Autodesk Inventor part; units mm, degrees
ref_plane "YZ Plane" through (0, 0, 0) normal (1, 0, 0) x (0, 1, 0)
ref_plane "XZ Plane" through (0, 0, 0) normal (0, 1, 0) x (-1, 0, 0)
ref_plane "XY Plane" through (0, 0, 0) normal (0, 0, 1) x (1, 0, 0)
sketch "Sketch1" plane through (0, 0, 0) normal (0, 0, 1) x (1, 0, 0)
  line L0 (0, 0) -> (150, 0)
  line L1 (150, 0) -> (150, 100)
  line L2 (150, 100) -> (0, 100)
  line L3 (0, 100) -> (0, 0)
  dimension "d0" = 150
  dimension "d1" = 100
extrude "Extrusion1" add sketch "Sketch1" along normal blind 250
fillet "Fillet1" radius 20 1 edges at (150, 100, 125)
fillet "Fillet2" radius 20 1 edges at (150, 0, 125)
fillet "Fillet3" radius 20 1 edges at (0, 100, 125)
fillet "Fillet4" radius 20 1 edges at (0, 0, 125)
fillet "Fillet5" radius 5 8 edges at (5.8579, 94.1421, 0) (0, 50, 0) (5.8579, 5.8579, 0) (75, 0, 0) (144.1421, 5.8579, 0) (150, 50, 0) (144.1421, 94.1421, 0) (75, 100, 0)
sketch "Sketch2" plane through (20, 0, 250) normal (0, -1, 0) x (1, 0, 0)
  line L0 (110, 0) -> (110, -245)
  line L1 (0, -245) -> (0, 0)
  line L2 (110, -171.6757) -> (0, -171.6757)
  line L3 (0, -171.6757) -> (0, -166.6757)
  line L4 (0, -166.6757) -> (110, -166.6757)
  line L5 (110, -166.6757) -> (110, -171.6757)
  line L6 (95.3863, -226.2308) -> (70.3863, -226.2308)
  line L7 (70.3863, -226.2308) -> (70.3863, -221.2308)
  line L8 (70.3863, -221.2308) -> (95.3863, -221.2308)
  line L9 (95.3863, -221.2308) -> (95.3863, -226.2308)
  line L10 (37.9599, -226.2308) -> (12.9599, -226.2308)
  line L11 (12.9599, -226.2308) -> (12.9599, -221.2308)
  line L12 (12.9599, -221.2308) -> (37.9599, -221.2308)
  line L13 (37.9599, -221.2308) -> (37.9599, -226.2308)
  line L14 (27.9599, -236.2308) -> (22.9599, -236.2308)
  line L15 (22.9599, -236.2308) -> (22.9599, -211.2308)
  line L16 (22.9599, -211.2308) -> (27.9599, -211.2308)
  line L17 (27.9599, -211.2308) -> (27.9599, -236.2308)
  point P0 (-20, -250)
  point P1 (27.9599, -226.2308)
  point P2 (27.9599, -221.2308)
  point P3 (22.9599, -221.2308)
  point P4 (22.9599, -226.2308)
  dimension "d9" = 25
  dimension "d10" = 5
  dimension "d11" = 5
  dimension "d12" = 25
  dimension "d13" = 10
  dimension "d14" = 10
  dimension "d15" = 5
  dimension "d16" = 25
  dimension "d17" = 5
extrude "Extrusion2" add sketch "Sketch2" along normal blind 5
sketch "Sketch3" plane through (0, 0, 0) normal (0, 0, -1) x (-1, 0, 0)
  line L0 (-20, 100) -> (-130, 100)
  line L1 (-150, 80) -> (-150, 20)
  circle A0 centre (-110, 50) radius 12.5
  circle A1 centre (-40, 51.4507) radius 12.5
  point P0 (0, 0)
  point P1 (-150, 50)
  dimension "d20" = 50
  dimension "d21" = 40
  dimension "d22" = 70
  dimension "d23" = 25
  dimension "d24" = 25
extrude "Extrusion3" add sketch "Sketch3" along normal blind 3
sketch "Sketch4" plane through (110, 50, -3) normal (0, 0, -1) x (-1, 0, 0)
  circle A0 centre (0, 0) radius 7.2404
  circle A1 centre (70, 1.4507) radius 12.5
  circle A2 centre (70, 1.4507) radius 7.5
  point P0 (110, -50)
  dimension "d27" = 15
extrude "Extrusion4" add sketch "Sketch4" along normal blind 15 contours A0 | A2
sketch "Sketch5" plane through (110, 50, -18) normal (0, 0, -1) x (-1, 0, 0)
  circle A0 centre (0, 0) radius 7.2404
  circle A1 centre (0, 0) radius 10
  circle A2 centre (70, 1.4507) radius 7.5
  circle A3 centre (70, 1.4507) radius 8.5
  point P0 (110, -50)
  dimension "d30" = 20
  dimension "d31" = 17
extrude "Extrusion5" add sketch "Sketch5" along normal blind 4 contours A0 | A1 | A2 | A3
sketch "Sketch6" plane through (110, 50, -22) normal (0, 0, -1) x (-1, 0, 0)
  circle A0 centre (0, 0) radius 10
  point P0 (110, -50)
hole "Hole1" at (110, 50, -22) direction (0, 0, 1) diameter 10.106 depth 28 tip angle 118
sketch "Sketch7" plane through (40, 51.4507, -22) normal (0, 0, -1) x (-1, 0, 0)
  circle A0 centre (0, 0) radius 8.5
  point P0 (40, -51.4507)
hole "Hole2" at (40, 51.4507, -22) direction (0, 0, 1) diameter 10.647 depth 28 tip angle 118
properties part number "battery eg 26"
The model under review builds one solid part; all positions refer to its coordinate system, in mm. A direction names the side the tool comes from. Coordinates: 2 decimals unless noted, no trailing zeros. Write each loop counter-clockwise with the first axis right and the second up, starting at its lowest first coordinate (ties: lowest second). Pieces come first, ordered by that corner, then holes.
1) Clearance check with flat-ended pins moving along their axes: pin 1 Ø8 at (x, z) = (68, 46.5) entering from -Y; pin 2 Ø4 at (x, y) = (101, -3.5) entering from -Z; pin 3 Ø1.5 at (y, z) = (-1.5, 25.5) entering from -X. State where each tip first meets the part, or that it passes through.
2) To check wall thickness, follow probe 1 along Y at (x, z) = (110, -0.75); probe 2 along Y at (x, z) = (40, -14); probe 3 along Z at (x, y) = (74, 24). State the ranges of each line that lie inside material, in increasing order.
3) The part is to be moulded in two halves that separate along Z. For faces 4 (the face through (104.6, 44.6, -3)), 5 (the face through (74, 0, 165)), 6 (the face through (53, -2, 23.769)), say which applies: pulls with the +Z half, pulls with the -Z half, needs draft (parallel to the pull), parting line crosses it, or undercut.
4) We need section A-A on z = 215. State the section outline as (x, y) points, then the cut area to 3 significant figures.
5) Machinability: for faces 1 (the face through (42.96, -2, 19)), 2 (the face through (53, -2, 28.769)), 3 (the face through (115.386, -2, 26)), which of the approach directions +Z, -Z, +X, -X, +Y, -Y give a long, thin tool a straight path to every point of the face, cutting with its end or side? Answer none if there is none.
Answer list:
1. pin 1: stops at y = 0
1. pin 2: stops at z = 23.77
1. pin 3: stops at x = 32.96
2. probe 1: y = 37.5 to 44.95, 55.05 to 62.5
2. probe 2: y = 43.95 to 46.13, 56.77 to 58.95
2. probe 3: z = 0 to 250
3. face 4: undercut
3. face 5: needs draft
3. face 6: pulls with the -Z half
4. outline: (0, 20) arc R20 ccw to (20, 0) - (130, 0) arc R20 ccw to (150, 20) - (150, 80) arc R20 ccw to (130, 100) - (20, 100) arc R20 ccw to (0, 80) - close
4. area: 14,700 mm2
5. face 1: -Z, -X, -Y
5. face 2: +X, -Y
5. face 3: -Z, +X, -Y
